from build123d import *

# Parameters (mm, degrees)
CROQUIS5_R              = 3
SALIENTE_EXTRUIR5_DEPTH = 28
ESCALA1_SCALE           = 7
ESCALA2_SCALE           = 7


with BuildPart() as part:
    # Croquis5 → Saliente-Extruir5 (new body)
    with BuildSketch(Plane.XY):
        Circle(CROQUIS5_R)
    extrude(amount=SALIENTE_EXTRUIR5_DEPTH)


with BuildPart() as part_1:
    # Escala1: scaled about (0, 0, 14)
    add(part.part.scale(ESCALA1_SCALE).moved(Location((0, 0, -84))))


with BuildPart() as part_2:
    # Escala2: scaled about (0, 0, 14)
    add(part_1.part.scale(ESCALA2_SCALE).moved(Location((0, 0, -84))))


solid = part_2.part
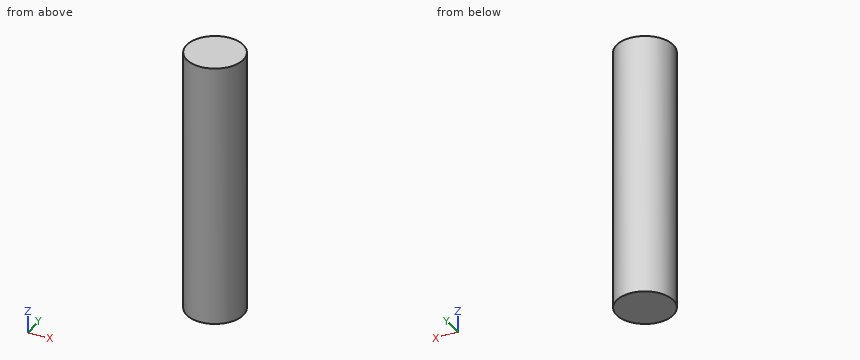
Source: CAD feature listing. Evaluate the final solid. Frame: model axes, mm. Give positions to 0.01 mm unless a question says otherwise; leave off trailing zeros. Write each loop counter-clockwise with the first axis right and the second up, starting at its lowest first coordinate (ties: lowest second). Pieces come first, ordered by that corner, then holes. Notation, with made-up numbers: M 70.25,-38.5 L 125.25,-38.5 A29 ccw 125.25,-18.5 Z; hole C 59.25,-40 d10. An arc over 180 degrees is marked long. Return JSON: item names as keys, results as strings. Group by question number.
1) Cut plane A-A, the plane z = 424. Output: boundary loops of the cut face in (x, y).
2) Cut plane C-C, the plane y = 38. Output: boundary loops of the cut face in (x, z).
3) Ray query, L1, parallel to X at y = -45, z = 312.5; L2, parallel to X at y = -74, z = 491.5; L3, parallel to Y at x = 14.5, z = 235. Return the intervals inside material, ascending.
4) Cut plane B-B, the plane x = 101. Output: boundary loops of the cut face in (y, z), then the cut area to 3 significant figures.
5) First-contact query: pin 1 Ø1 at (x, z) = (-61.5, -56.5) entering from -Y; pin 2 Ø1.5 at (x, z) = (-20, -271) entering from +Y; pin 3 Ø3 at (y, z) = (106.5, -246.5) entering from -X. Flat tips, straight axial feed; report the tip coordinate or a pass-through.
Data:
{
 "1": {"outline": "C 0,0 d294"},
 "2": {"outline": "M -142,-672 L 142,-672 L 142,700 L -142,700 Z"},
 "3": {"L1": "x = -139.94 to 139.94", "L2": "x = -127.02 to 127.02", "L3": "y = -146.28 to 146.28"},
 "4": {"outline": "M -106.81,-672 L 106.81,-672 L 106.81,700 L -106.81,700 Z", "area": "293,000 mm²"},
 "5": {"pin 1": "stops at y = -133.75", "pin 2": "stops at y = 145.73", "pin 3": "stops at x = -102.88"}
}
